The model under review builds one solid part; all positions refer to its coordinate system, in mm. Face numbers are marked on the shaded views. A direction names the side the tool comes from. Give positions to 0.01 mm unless a question says otherwise; leave off trailing zeros. Write each loop counter-clockwise with the first axis right and the second up, starting at its lowest first coordinate (ties: lowest second). Pieces come first, ordered by that corner, then holes. Notation, with made-up numbers: (34, 17) - (77, 17) arc R25 cw to (77, 48) - close; hole circle Ø10 at (44.5, -36.5). An arc over 180 degrees is marked (long way). Write item = value, one per line.
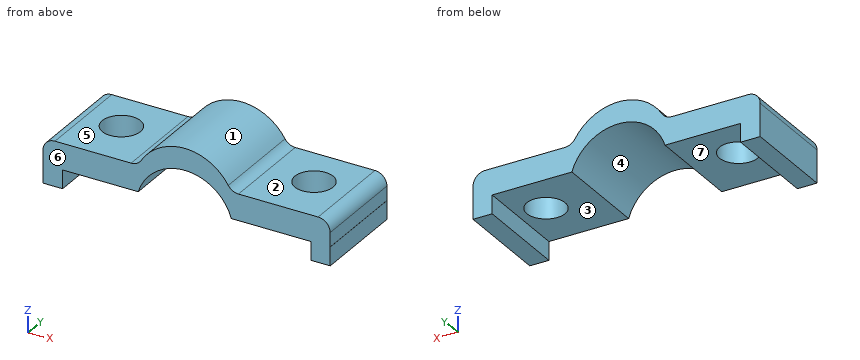
```python
from build123d import *

# Parameters (mm, degrees)
F1_DEPTH = 50.8
F3_D     = 20.32


with BuildPart() as f1:
    # F0 (on Front) → F1 (new body)
    with BuildSketch(Plane.XZ):
        with BuildLine():
            ThreePointArc((-25.6362788903, 0), (-0.9451183533, 18.1852056191), (23.7460421838, 0))
            Line((23.7460421838, 0), (66.0344064236, 0))
            Line((66.0344064236, 0), (66.0344064236, -9.8256887868))
            Line((66.0344064236, -9.8256887868), (76.2, -9.8256887868))
            Line((76.2, -9.8256887868), (76.2, 0))
            Line((76.2, 0), (76.149083674, 0))
            Line((76.149083674, 0), (76.149083674, 7.5215598732))
            ThreePointArc((76.149083674, 7.5215598732), (74.2892117345, 12.0116879338), (69.799083674, 13.8715598732))
            Line((69.799083674, 13.8715598732), (27.5173505631, 13.8715598732))
            ThreePointArc((27.5173505631, 13.8715598732), (24.4377427448, 14.6683161648), (22.1309528492, 16.8586415471))
            ThreePointArc((22.1309528492, 16.8586415471), (-0.9451183533, 29.6557116959), (-24.0211895558, 16.8586415471))
            ThreePointArc((-24.0211895558, 16.8586415471), (-26.3279794513, 14.6683161648), (-29.4075872696, 13.8715598732))
            Line((-29.4075872696, 13.8715598732), (-69.799083674, 13.8715598732))
            ThreePointArc((-69.799083674, 13.8715598732), (-74.2892117345, 12.0116879338), (-76.149083674, 7.5215598732))
            Line((-76.149083674, 7.5215598732), (-76.149083674, 0))
            Line((-76.149083674, 0), (-76.149083674, -9.8256887868))
            Line((-76.149083674, -9.8256887868), (-65.7454133034, -9.8256887868))
            Line((-65.7454133034, -9.8256887868), (-65.7454133034, 0))
            Line((-65.7454133034, 0), (-25.6362788903, 0))
        make_face()
    extrude(amount=F1_DEPTH)

    # F3 (through all)
    with Locations(Plane(origin=(0, 0, 0), x_dir=(1, 0, 0), z_dir=(0, 0, -1))):
        with Locations((-50.9421490133, 23.1955610216), (51.2357614934, 23.1955610216)):
            Hole(F3_D / 2)


solid = f1.part
```
1. Take a section at B-B on x = 50.5. Give the boundary of the cut face in (y, z).
Findings below:
outline = (-50.8, 0) - (-33.33, 0) - (-33.33, 13.87) - (-50.8, 13.87) - close; (-13.06, 0) - (0, 0) - (0, 13.87) - (-13.06, 13.87) - close
2. Insertion check: P1, Ø10, axis at x = -42, y = -39, coming from the -Z side; P2, Ø12, axis at x = -50.94, y = -23.2, coming from the +Z side; P3, Ø3, axis at x = -7, y = -35.5, coming from the -Z side; P4, Ø23.5, axis at x = 51.24, y = -23.2, coming from the +Z side. Each pin has a flat end and moves straight along its axis. Give the tip position at first contact, or say it passes through.
Findings below:
P1 = 0
P2 = through
P3 = 17.06
P4 = 13.87
3. Take a section at D-D on y = -36.5. Give the boundary of the cut face in (x, z).
Findings below:
outline = (-76.15, -9.83) - (-65.75, -9.83) - (-65.75, 0) - (-25.64, 0) arc R25.85 cw to (23.75, 0) - (66.03, 0) - (66.03, -9.83) - (76.2, -9.83) - (76.2, 0) - (76.15, 0) - (76.15, 7.52) arc R6.35 ccw to (69.8, 13.87) - (27.52, 13.87) arc R6.35 cw to (22.13, 16.86) arc R27.2 ccw to (-24.02, 16.86) arc R6.35 cw to (-29.41, 13.87) - (-69.8, 13.87) arc R6.35 ccw to (-76.15, 7.52) - close
4. For line 1 (X direction, y = -37.5, z = -4); line 2 (Z direction, x = -70, y = -19.5); line 3 (X direction, y = -8, z = 11), list the stretches that pass through material, from the lowest coordinate up. Write a range as from..to.
Findings below:
line_1 = -76.15..-65.75, 66.03..76.2
line_2 = -9.83..13.87
line_3 = -75.11..-18.83, 16.94..75.11
5. Draft analysis for pull direction X (two halves, no side actions). For the marked faces 1, 2, 3 and 4, state which applies: +X half, -X half, draft (parallel to the pull), parting line (faces both ways), or undercut.
Findings below:
face_1 = parting line
face_2 = draft
face_3 = undercut
face_4 = undercut
6. Take a section at A-A on z = -6. Give the boundary of the cut face in (x, y).
Findings below:
outline = (-76.15, -50.8) - (-65.75, -50.8) - (-65.75, 0) - (-76.15, 0) - close; (66.03, -50.8) - (76.2, -50.8) - (76.2, 0) - (66.03, 0) - close
7. Take a section at C-C on z = 10. Give the boundary of the cut face in (x, y), and give its area (3 significant figures).
Findings below:
outline = (-75.65, -50.8) - (-19.82, -50.8) - (-19.82, 0) - (-75.65, 0) - close; (17.93, -50.8) - (75.65, -50.8) - (75.65, 0) - (17.93, 0) - close; hole circle Ø20.32 at (-50.94, -23.2); hole circle Ø20.32 at (51.24, -23.2)
area = 5,120 mm²
8. Machinability: for the marked faces 5, 6 and 7, which of the approach directions +Z, -Z, +X, -X, +Y, -Y give a long, thin tool a straight path to every point of the face, cutting with its end or side? Answer none if there is none.
Findings below:
face_5 = +Z, -X, +Y, -Y
face_6 = +Z, -Z, +X, -X, -Y
face_7 = -Z, +Y, -Y
